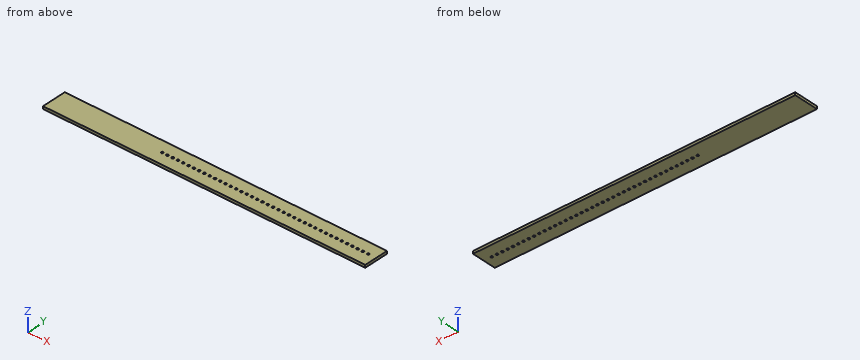
from build123d import *

# Parameters (mm, degrees)
SKETCH_1_W             = 1220
SKETCH_1_H             = 94
EXTRUDE_1_DEPTH        = 10
MM_1_D                 = 8
PATTERN_LINEAR_1_COUNT = 40
PATTERN_LINEAR_1_PITCH = 20


with BuildPart() as part:
    # 草图1 → 凸台-拉伸1 (new body)
    with BuildSketch(Plane.XY):
        Rectangle(SKETCH_1_W, SKETCH_1_H)
    extrude(amount=EXTRUDE_1_DEPTH)

    # 大小mm 暗销孔1 (through all)
    with Locations(Plane(origin=(0, 0, 0), x_dir=(-1, 0, 0), z_dir=(0, 0, -1))):
        with Locations((-580, 0)):
            mm_1 = Hole(MM_1_D / 2)

    # 阵列(线性)1: 大小mm 暗销孔1 ×40
    with Locations(*[(-i * PATTERN_LINEAR_1_PITCH, 0, 0) for i in range(1, PATTERN_LINEAR_1_COUNT)]):
        add(mm_1, mode=Mode.SUBTRACT)


solid = part.part
Check sheet for the modelled part. Datum: model origin and axes. Units: mm. Give positions to 0.01 mm unless a question says otherwise; leave off trailing zeros. Use one line per item in the form item = value.
(1) Depth check by flat-ended pin: P1, Ø13, axis at x = 500, y = 0, coming from the +Z side. Enter the tip coordinate at first touch or a pass-through.
Answer block:
P1 = 10
(2) Section check A-A on z = 6.25. State how many separate pieces and enclosed holes the cut face has, plus the area to 3 significant figures.
Answer block:
separate_pieces = 1
enclosed_holes = 40
area = 113,000 mm2
(3) Material ranges on line 1 along Y through (x, z) = (40, 8); line 2 along Y through (x, z) = (-163, 5.5), recorded low to high.
Answer block:
line_1 = -47 to -4, 4 to 47
line_2 = -47 to -2.65, 2.65 to 47
